Autodesk Inventor part; units mm, degrees
ref_plane "YZ Plane" through (0, 0, 0) normal (1, 0, 0) x (0, 1, 0)
ref_plane "XZ Plane" through (0, 0, 0) normal (0, 1, 0) x (-1, 0, 0)
ref_plane "XY Plane" through (0, 0, 0) normal (0, 0, 1) x (1, 0, 0)
sketch "草图1" plane through (0, 0, 0) normal (0, 0, 1) x (1, 0, 0)
  line L0 (-40, 0) -> (40, 0)
  line L1 (40, 0) -> (40, 5)
  line L2 (40, 5) -> (-40, 5)
  line L3 (-40, 5) -> (-40, 0)
  arc A0 (26, 0) -> (-26, 0) centre (0, 0) ccw
  dimension "d0" = 80
  dimension "d1" = 5
  dimension "d2" = 26
extrude "拉伸1" add sketch "草图1" along normal blind 14
sketch "草图2" plane through (0, 0, 14) normal (0, 0, 1) x (1, 0, 0)
  circle A0 centre (0, 0) radius 21
  dimension "d5" = 42
extrude "拉伸2" cut sketch "草图2" against normal blind 7
sketch "草图3" plane through (0, 0, 7) normal (0, 0, 1) x (1, 0, 0)
  circle A0 centre (0, 0) radius 17
  dimension "d8" = 34
extrude "拉伸3" cut sketch "草图3" against normal blind 2
sketch "草图4" plane through (0, 0, 5) normal (0, 0, 1) x (1, 0, 0)
  circle A0 centre (0, 0) radius 15.5
  dimension "d11" = 31
extrude "拉伸4" cut sketch "草图4" against normal blind 5
sketch "草图5" plane through (-40, 5, 0) normal (0, 1, 0) x (1, 0, 0)
  circle A0 centre (7, -7) radius 2.5
  circle A1 centre (73, -7) radius 2.5
  line L0 (80, 0) -> (80, -14)
  line L1 (80, -14) -> (65.5147, -14)
  line L2 (0, 0) -> (0, -14)
  line L3 (14.4853, -14) -> (0, -14)
  point P0 (40, 0)
  dimension "d14" = 5
  dimension "d15" = 5
  dimension "d16" = 7
  dimension "d17" = 7
  dimension "d18" = 7
  dimension "d19" = 7
extrude "拉伸5" cut sketch "草图5" against normal through all
properties part number "电机座上轴盖"
Can you work these out from the model? Positions are in its coordinate system, mm. A direction names the side the tool comes from. Coordinates: 2 decimals unless noted, no trailing zeros. Loops run counter-clockwise (first coordinate to the right, second up) from the corner with the lowest first, then second, coordinate; pieces in that order, holes last.
1) Which directions (+Z, -Z, +X, -X, +Y, -Y) give clear straight access to the entire face, cutting with the end or side of a thin tool? Please do faces 1 (the flat face through (33, 5, 10)), 2 (the flat face through (0, 22, 14)), 3 (the cylindrical face through (0, 21, 11)).
2) Imagine slicing it at B-B on z = 2. List the corners of the cut face in (x, y) for me, plus the area to 3 significant figures.
3) Imagine slicing it at D-D on x = 0. List the corners of the cut face in (y, z) for me.
4) Thinking about a two-plate mould opening in Z: for faces 4 (the flat face through (-1, 16, 0)), 5 (the flat face through (-31, 5, 5)), 6 (the cylindrical face through (-35.5, 2.5, 6.9)), 7 (the flat face through (2.4, 15.5, 5)), which applies, pulls with the +Z half, pulls with the -Z half, needs draft (parallel to the pull), parting line crosses it, or undercut?
5) Imagine slicing it at A-A on x = -33. List the corners of the cut face in (y, z) for me.
6) For pin 1 (10.5 mm diameter, centred on x = 0.5, y = 13, fed in from +Z); pin 2 (4.5 mm diameter, centred on x = 33, z = 7, fed in from +Y); pin 3 (4 mm diameter, centred on x = 34.5, z = 7.5, fed in from +Y); pin 4 (6 mm diameter, centred on y = 11, z = 5, fed in from +X), each with a flat end and sliding along its axis, tell me the tip position at first contact or that it passes through.
7) Imagine slicing it at C-C on y = 12.5. List the corners of the cut face in (x, z) for me, plus the area to 3 significant figures.
8) I need wall thicknesses on probe 1 along Z at (x, y) = (33, 3.2); probe 2 along Z at (x, y) = (14, 13.25); probe 3 along Y at (x, z) = (27, 7.25). Which ranges of each line are inside material? Lowest first, please.
Completed:
1. face 1: +Z, -Z, +X, +Y
1. face 2: +Z, +X, -X, +Y, -Y
1. face 3: +Z, -Y
2. outline: (-40, 0) - (-15.5, 0) arc R15.5 cw to (15.5, 0) - (40, 0) - (40, 5) - (25.51, 5) arc R26 ccw to (-25.51, 5) - (-40, 5) - close
2. area: 826 mm2
3. outline: (15.5, 0) - (26, 0) - (26, 14) - (21, 14) - (21, 7) - (17, 7) - (17, 5) - (15.5, 5) - close
4. face 4: pulls with the -Z half
4. face 5: needs draft
4. face 6: undercut
4. face 7: pulls with the +Z half
5. outline: (0, 0) - (5, 0) - (5, 4.5) - (0, 4.5) - close; (0, 9.5) - (5, 9.5) - (5, 14) - (0, 14) - close
6. pin 1: stops at z = 7
6. pin 2: passes through
6. pin 3: stops at y = 5
6. pin 4: stops at x = 24.74
7. outline: (-22.8, 0) - (-9.17, 0) - (-9.17, 5) - (-11.52, 5) - (-11.52, 7) - (-16.87, 7) - (-16.87, 14) - (-22.8, 14) - close; (9.17, 0) - (22.8, 0) - (22.8, 14) - (16.87, 14) - (16.87, 7) - (11.52, 7) - (11.52, 5) - (9.17, 5) - close
7. area: 264 mm2
8. probe 1: z = 0 to 4.5, 9.5 to 14
8. probe 2: z = 0 to 7
8. probe 3: y = 0 to 5
